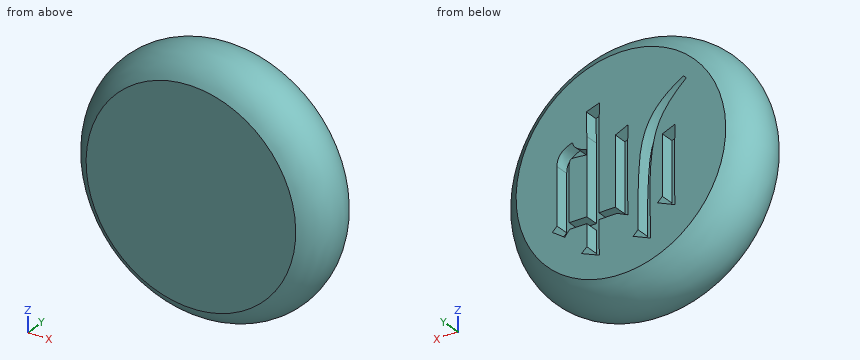
from build123d import *

# Parameters (mm, degrees)
CUT_EXTRUDE_1_DEPTH = 2


with BuildPart() as part:
    # 草图1 → 旋转1 (revolve)
    with BuildSketch(Plane.XY, mode=Mode.PRIVATE) as revolve_1_sk:
        with BuildLine():
            Line((0, 0), (15, 0))
            ThreePointArc((15, 0), (18, 5), (15, 10))
            Line((15, 10), (0, 10))
            Line((0, 10), (0, 0))
        make_face()
    revolve(revolve_1_sk.sketch.rotate(Axis((0, 13.411477292, 0), (0, -1, 0)), 90), axis=Axis((0, 13.411477292, 0), (0, -1, 0)))

    # 草图3 → 切除-拉伸1 (cut)
    with BuildSketch(Plane(origin=(0, 10, 0), x_dir=(1, 0, 0), z_dir=(0, 1, 0))):
        with BuildLine():
            add(Edge.make_bspline(
                [(-7.737435646, -2.797446042), (-7.731068719, -2.587685086), (-7.717945409, -2.155332343), (-7.696642932, -1.488687912), (-7.686423073, -0.784380082), (-7.672167654, -0.044911976), (-7.662660109, 0.731003875), (-7.657710892, 1.542239007), (-7.648610401, 2.390894981), (-7.65186825, 3.256706013), (-7.648559979, 4.1032554), (-7.65746445, 4.891980565), (-7.662502543, 5.604758223), (-7.671605944, 6.241565546), (-7.685936074, 6.8022931), (-7.695789632, 7.287287836), (-7.716164539, 7.694960994), (-7.730854842, 7.941006207), (-7.737435646, 8.051226903)],
                knots=[0, 0, 0, 0, 0.928317114, 1.913418291, 2.950357829, 4.044097515, 5.185102596, 6.382865837, 7.632702554, 8.939312537, 10.212783862, 11.377409509, 12.428421057, 13.365879284, 14.194562146, 14.909661131, 15.511561687, 16, 16, 16, 16], degree=3))
            Line((-7.737435646, 8.051226903), (-5.249207906, 7.020619026))
            Line((-5.249207906, 7.020619026), (-5.929858591, 6.349600191))
            Line((-5.929858591, 6.349600191), (-5.929858591, -2.059004261))
            Line((-5.929858591, -2.059004261), (-7.737435646, -2.797446042))
        make_face()
        with BuildLine():
            add(Edge.make_bspline(
                [(-9.352375714, -8.534817617), (-9.084525015, -8.300974918), (-8.562369969, -7.845115942), (-7.839466918, -7.133926567), (-7.190646214, -6.425865151), (-6.614868907, -5.721727451), (-6.117599742, -5.01766043), (-5.699034732, -4.312825243), (-5.35196567, -3.611575818), (-5.078196611, -2.899933759), (-4.858394528, -2.160239778), (-4.674985415, -1.371412367), (-4.513140358, -0.524594418), (-4.388643582, 0.382421036), (-4.283467988, 1.346814475), (-4.217243739, 2.370936396), (-4.169114628, 3.45422046), (-4.163132935, 4.574135062), (-4.162447067, 5.68500678), (-4.170367209, 6.74022891), (-4.177021693, 7.717319618), (-4.181368154, 8.616338485), (-4.194730299, 9.437192973), (-4.211775037, 10.179872076), (-4.226060685, 10.843485892), (-4.240662817, 11.259714785), (-4.247495577, 11.454480328)],
                knots=[0, 0, 0, 0, 1.185402125, 2.310853403, 3.379298985, 4.386389788, 5.341776688, 6.250603628, 7.117198236, 7.947562309, 8.789765669, 9.688220653, 10.647060204, 11.663458785, 12.7400909, 13.881155971, 15.084787921, 16.355264848, 17.614955996, 18.789024112, 19.873880758, 20.873094693, 21.786749924, 22.611273472, 23.350174675, 24, 24, 24, 24], degree=3))
            Line((-4.247495577, 11.454480328), (-1.759267838, 10.430293684))
            Line((-1.759267838, 10.430293684), (-2.446339755, 9.756064232))
            add(Edge.make_bspline(
                [(-2.446339755, 9.756064232), (-2.440091603, 9.296954134), (-2.427886973, 8.400166089), (-2.425054866, 7.088026543), (-2.433852361, 5.841156766), (-2.457190325, 4.659621552), (-2.487940385, 3.542189591), (-2.532130363, 2.488939398), (-2.591199959, 1.501176574), (-2.654809669, 0.574553083), (-2.745066202, -0.298269112), (-2.877247045, -1.122116359), (-3.041703355, -1.903705624), (-3.251953741, -2.638406345), (-3.493159764, -3.332378276), (-3.78089571, -3.978119394), (-4.100727381, -4.582126813), (-4.465575897, -5.142882654), (-4.871083747, -5.674414465), (-5.322135975, -6.183582916), (-5.815645595, -6.680645685), (-6.355725979, -7.162346781), (-6.944200864, -7.627281526), (-7.57898216, -8.076065119), (-8.255596092, -8.514663533), (-8.73132227, -8.785443356), (-8.973522975, -8.923302207)],
                knots=[0, 0, 0, 0, 1.560783084, 3.048705779, 4.460269439, 5.799274246, 7.065800622, 8.260132026, 9.382529971, 10.429410577, 11.417304408, 12.364078358, 13.264555336, 14.130553639, 14.960140012, 15.759842068, 16.531300228, 17.281042902, 18.03120911, 18.801912066, 19.591647171, 20.410984061, 21.260379231, 22.139595362, 23.052834729, 24, 24, 24, 24], degree=3))
            Line((-8.973522975, -8.923302207), (-9.352375714, -8.534817617))
        make_face()
        with BuildLine():
            add(Edge.make_bspline(
                [(3.152975313, 6.622502588), (3.153588126, 6.89540738), (3.154770514, 7.421962128), (3.146611659, 8.180724822), (3.140028092, 8.877422102), (3.135631354, 9.512118402), (3.122401095, 10.084693336), (3.105340851, 10.596188458), (3.091104619, 11.045807919), (3.076344341, 11.325003722), (3.069499286, 11.454480328)],
                knots=[0, 0, 0, 0, 1.355131449, 2.614651405, 3.767890675, 4.814850097, 5.76633671, 6.611718708, 7.356186779, 8, 8, 8, 8], degree=3))
            Line((3.069499286, 11.454480328), (5.641203053, 10.420661835))
            Line((5.641203053, 10.420661835), (4.87707634, 9.743221766))
            Line((4.87707634, 9.743221766), (4.87707634, 6.622502588))
            Line((4.87707634, 6.622502588), (7.336408532, 6.622502588))
            Line((7.336408532, 6.622502588), (8.036322916, 7.473315944))
            Line((8.036322916, 7.473315944), (9.811793806, 6.253281698))
            Line((9.811793806, 6.253281698), (9.131143121, 5.617579643))
            Line((9.131143121, 5.617579643), (9.131143121, -2.399329604))
            add(Edge.make_bspline(
                [(9.131143121, -2.399329604), (9.131395669, -2.546397527), (9.131885996, -2.831932311), (9.038977853, -3.246324843), (8.869656202, -3.623256102), (8.626107599, -3.965580357), (8.304608549, -4.264870746), (7.911665558, -4.529495739), (7.446925145, -4.762008048), (7.102712639, -4.875966944), (6.922239012, -4.93571659)],
                knots=[0, 0, 0, 0, 0.96219561, 1.868118553, 2.760343656, 3.656205337, 4.604451048, 5.624548914, 6.75453022, 8, 8, 8, 8], degree=3))
            add(Edge.make_bspline(
                [(6.922239012, -4.93571659), (6.909123756, -4.854277288), (6.882545497, -4.689239347), (6.76543208, -4.457080757), (6.597014494, -4.239577573), (6.375934205, -4.032062925), (6.094335298, -3.845055724), (5.760972018, -3.665348344), (5.3728269, -3.494916639), (5.089884589, -3.401790672), (4.941288669, -3.352882686)],
                knots=[0, 0, 0, 0, 0.736733597, 1.493001439, 2.301925965, 3.199030657, 4.20096543, 5.327273661, 6.596334963, 8, 8, 8, 8], degree=3))
            Line((4.941288669, -3.352882686), (4.941288669, -2.652968302))
            add(Edge.make_bspline(
                [(4.941288669, -2.652968302), (5.067580967, -2.665728809), (5.309464653, -2.690168608), (5.652829722, -2.726155562), (5.961218582, -2.754387456), (6.23180788, -2.780889296), (6.468341952, -2.800346265), (6.66736422, -2.813966281), (6.831367995, -2.818966606), (6.961738085, -2.825714194), (7.073934615, -2.817350678), (7.1666596, -2.768928995), (7.242752738, -2.694357526), (7.305466829, -2.593339306), (7.350603643, -2.463928678), (7.386512175, -2.307952974), (7.403655814, -2.123586173), (7.405861386, -1.99160248), (7.407042094, -1.920947754)],
                knots=[0, 0, 0, 0, 1.935290813, 3.70660193, 5.263620808, 6.65666223, 7.851791597, 8.881808183, 9.698291315, 10.351159825, 10.877354834, 11.388145665, 11.907465341, 12.486877492, 13.183923572, 13.987423657, 14.922609108, 16, 16, 16, 16], degree=3))
            Line((7.407042094, -1.920947754), (7.407042094, 5.70105567))
            Line((7.407042094, 5.70105567), (4.87707634, 5.70105567))
            Line((4.87707634, 5.70105567), (4.87707634, -5.12514296))
            add(Edge.make_bspline(
                [(4.87707634, -5.12514296), (4.880062675, -5.679591911), (4.886054434, -6.792034181), (4.933528892, -7.903479956), (4.957341751, -8.460973439)],
                knots=[0, 0, 0, 0, 0.996813886, 2, 2, 2, 2], degree=3))
            Line((4.957341751, -8.460973439), (3.069499286, -9.093464878))
            add(Edge.make_bspline(
                [(3.069499286, -9.093464878), (3.076173355, -8.874079729), (3.089227829, -8.444962546), (3.104114646, -7.815620094), (3.12099665, -7.214217278), (3.135029943, -6.640611688), (3.139755388, -6.093672162), (3.145931121, -5.574624741), (3.154576391, -5.083429325), (3.153498098, -4.765557311), (3.152975313, -4.61144433)],
                knots=[0, 0, 0, 0, 1.175035445, 2.298368424, 3.370154139, 4.395977557, 5.370047505, 6.298285367, 7.17496255, 8, 8, 8, 8], degree=3))
            Line((3.152975313, -4.61144433), (3.152975313, 5.70105567))
            Line((3.152975313, 5.70105567), (0.793172231, 5.70105567))
            Line((0.793172231, 5.70105567), (0.793172231, -4.020690905))
            Line((0.793172231, -4.020690905), (-1.014404824, -4.849029946))
            add(Edge.make_bspline(
                [(-1.014404824, -4.849029946), (-1.00758523, -4.672458776), (-0.993121685, -4.297972388), (-0.978711974, -3.703916925), (-0.961773948, -3.046857597), (-0.948257418, -2.325535215), (-0.943934204, -1.541021297), (-0.937399912, -0.69128389), (-0.928883861, 0.221590297), (-0.931985888, 1.178367317), (-0.928877241, 2.136214544), (-0.93744001, 3.054439424), (-0.943919928, 3.911668811), (-0.948313778, 4.707953238), (-0.961785981, 5.443188246), (-0.978767285, 6.117371114), (-0.993218695, 6.730684991), (-1.007592937, 7.119089948), (-1.014404824, 7.303153273)],
                knots=[0, 0, 0, 0, 0.697843585, 1.480043001, 2.346745801, 3.293646528, 4.329188613, 5.445032886, 6.649632591, 7.934507307, 9.223608584, 10.432434748, 11.560958345, 12.609179698, 13.577209938, 14.465039412, 15.272589231, 16, 16, 16, 16], degree=3))
            Line((-1.014404824, 7.303153273), (0.526691066, 6.622502588))
            Line((0.526691066, 6.622502588), (3.152975313, 6.622502588))
        make_face()
    extrude(amount=-CUT_EXTRUDE_1_DEPTH, mode=Mode.SUBTRACT)


solid = part.part
CAD build for the part. Positions are in the model's coordinates, mm. Round coordinates to 2 decimals unless told otherwise and drop trailing zeros. Order: outer loops, then holes, each group sorted by start corner. A loop starts at its lowest first (then second) coordinate and runs counter-clockwise, first axis right, second up. Notation, with made-up numbers: (30, 48.5) - (45, 48.5) arc R7 ccw to (45, 56.5) - close; hole circle Ø9 at (34.5, -33). An arc over 180 degrees is marked (long way). Return JSON: item names as keys, results as strings.
(1) Pin check, flat tips, straight feed: pin 1 Ø0.6 at (y, z) = (9.5, 0) entering from -X; pin 2 Ø1.6 at (y, z) = (9.5, 0) entering from +X; pin 3 Ø2 at (x, y) = (6, 8.5) entering from -Z. Stop position of each tip, or through.
Answer key:
{"pin 1": "stops at x = -16.14", "pin 2": "stops at x = 16.63", "pin 3": "stops at z = -16.46"}
(2) Cut at B-B (y = 3). Give the cut face in (x, z), then the cut area to 3 significant figures.
Answer key:
{"outline": "circle Ø35.27 at (0, 0)", "area": "977 mm^2"}
(3) Cut at A-A (y = 5.5). Give the cut face in (x, z).
Answer key:
{"outline": "circle Ø35.96 at (0, 0)"}
(4) Wall check: probe 1 along X at (y, z) = (9.75, 1); probe 2 along X at (y, z) = (9.75, -3); probe 3 along Z at (x, y) = (-6, 9). Give the ranges that are in metal, low to high. Write a range as from..to.
Answer key:
{"probe 1": "x = -15.39..-7.69, -5.93..-4.61, -2.86..-0.94, 0.79..3.15, 4.88..7.41, 9.13..15.39", "probe 2": "x = -15.13..-7.65, -5.93..-4.19, -2.51..-0.94, 0.79..3.15, 4.88..7.41, 9.13..15.13", "probe 3": "z = -15.21..-7.33, 2.09..4.81, 6.84..15.21"}
